Input: dimensioned drawing with shaded views. Units: mm. Origin: part minimum x, y, z. Round coordinates to 2 decimals unless told otherwise and drop trailing zeros. Loops run counter-clockwise (first coordinate to the right, second up) from the corner with the lowest first, then second, coordinate; pieces in that order, holes last. Notation, with made-up numbers: (46, -24.75) -> (79, -24.75) arc R22 cw to (79, 12.25) -> close; hole circle Ø6 at (-3.5, 75). An arc over 180 degrees is marked (long way). Answer as a JSON object with one key per item and string values.
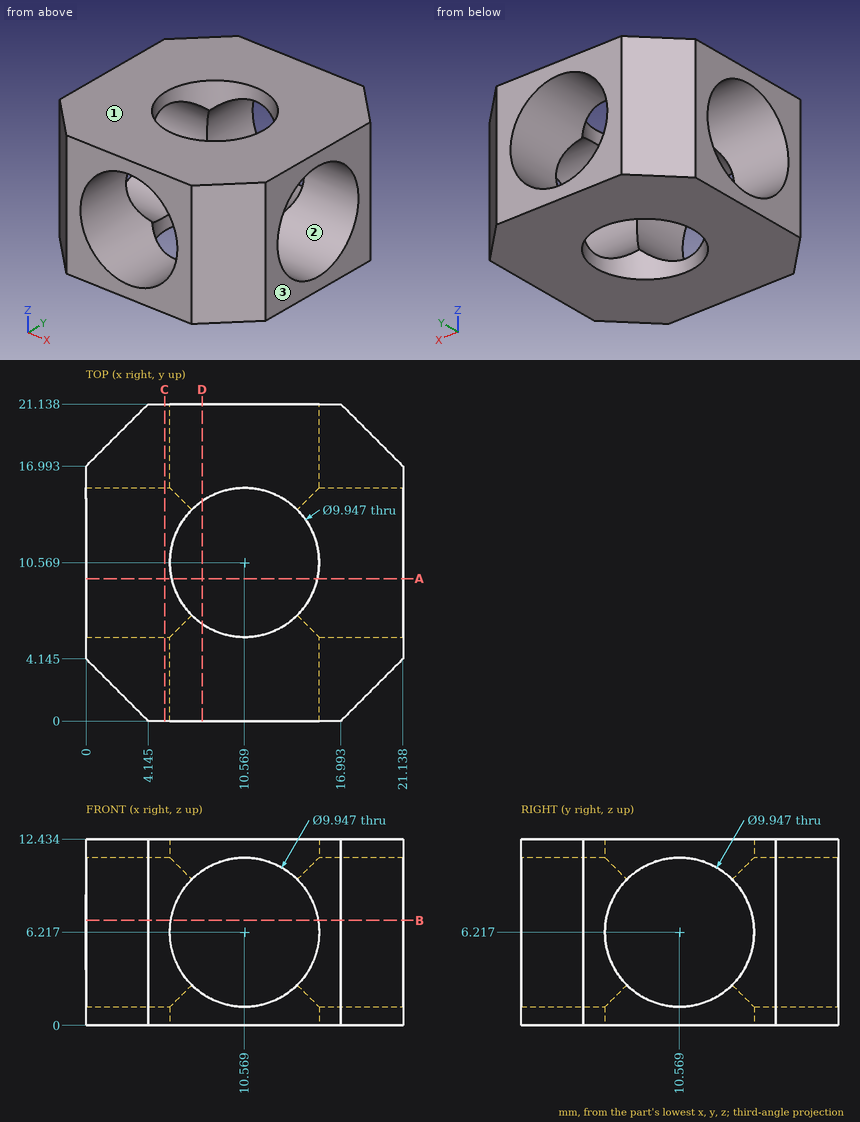
1) Ray query, probe 1 along Y at (x, z) = (10.75, 11.25); probe 2 along Z at (x, y) = (5, 10.75) (1 decimal); probe 3 along Z at (x, y) = (16.25, 12.25) (1 decimal). Return the intervals inside material, ascending.
Output:
{"probe 1": "y = 0 to 5.6, 15.54 to 21.14", "probe 2": "z = 0 to 1.2, 11.2 to 12.4", "probe 3": "z = 0 to 1.5, 10.9 to 12.4"}
2) Section C-C, the plane x = 5.25. Output: boundary loops of the cut face in (y, z) (1 decimal), plus the area to 3 significant figures.
Output:
{"outline": "(0, 0) -> (21.1, 0) -> (21.1, 12.4) -> (0, 12.4) -> close; hole circle Ø9.9 at (10.6, 6.2)", "area": "185 mm^2"}
3) Draft query along Z for the marked faces 1, 2 and 3. Return one class per face: +Z half, -Z half, draft (parallel to the pull), parting line (faces both ways), or undercut.
Output:
{"face 1": "+Z half", "face 2": "undercut", "face 3": "draft"}
4) Section B-B, the plane z = 7. Output: boundary loops of the cut face in (x, y) (1 decimal).
Output:
{"outline": "(0, 4.1) -> (4.1, 0) -> (5.7, 0) -> (5.7, 5.7) -> (0, 5.7) -> close; (0, 15.5) -> (5.7, 15.5) -> (5.7, 21.1) -> (4.1, 21.1) -> (0, 17) -> close; (15.5, 0) -> (17, 0) -> (21.1, 4.1) -> (21.1, 5.7) -> (15.5, 5.7) -> close; (15.5, 15.5) -> (21.1, 15.5) -> (21.1, 17) -> (17, 21.1) -> (15.5, 21.1) -> close"}
5) Section D-D, the plane x = 7.75. Output: boundary loops of the cut face in (y, z) (1 decimal).
Output:
{"outline": "(0, 0) -> (6.5, 0) -> (6.5, 2.1) -> (0, 2.1) -> close; (0, 10.3) -> (6.5, 10.3) -> (6.5, 12.4) -> (0, 12.4) -> close; (14.7, 0) -> (21.1, 0) -> (21.1, 2.1) -> (14.7, 2.1) -> close; (14.7, 10.3) -> (21.1, 10.3) -> (21.1, 12.4) -> (14.7, 12.4) -> close"}
6) Section A-A, the plane y = 9.5. Output: boundary loops of the cut face in (x, z) (1 decimal).
Output:
{"outline": "(0, 0) -> (5.7, 0) -> (5.7, 1.4) -> (0, 1.4) -> close; (0, 11.1) -> (5.7, 11.1) -> (5.7, 12.4) -> (0, 12.4) -> close; (15.4, 0) -> (21.1, 0) -> (21.1, 1.4) -> (15.4, 1.4) -> close; (15.4, 11.1) -> (21.1, 11.1) -> (21.1, 12.4) -> (15.4, 12.4) -> close"}
7) Contact query for a flat-ended pin moving along its axis: P1, Ø1, axis at x = 7, z = 7.5, coming from the -Y side. Output: stop coordinate, or through.
Output:
{"P1": "passes through"}
